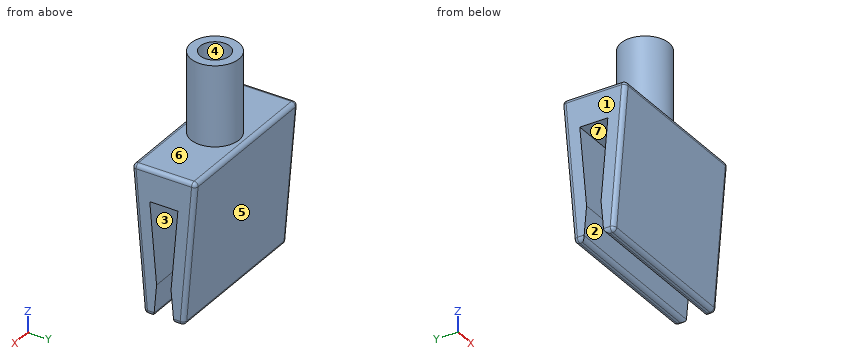
```python
from build123d import *

# Parameters (mm, degrees)
F1_DEPTH = 10
F3_DEPTH = 25
F4_R     = 0.5
F5_R     = 3
F5_R_2   = 1.85
F6_DEPTH = 10


with BuildPart() as f1:
    # F0 (on Right) → F1 (new body, symmetric)
    with BuildSketch(Plane.YZ):
        Polygon((-45.5818854975, 27.2887923438), (-44.0818854975, 9.2887923438), (-39.0818854975, 9.2887923438), (-37.5818854975, 27.2887923438), align=None)
    extrude(amount=F1_DEPTH, both=True)

    # F2 (on face) → F3 (cut)
    with BuildSketch(Plane.YZ.offset(10)):
        Polygon((-42.8318854975, 9.2887923438), (-40.3318854975, 9.2887923438), (-40.6818854975, 13.2887923438), (-39.8318854975, 23.2887923438), (-41.5818854975, 23.2887923438), (-43.3318854975, 23.2887923438), (-42.4818854975, 13.2887923438), align=None)
    extrude(amount=-F3_DEPTH, mode=Mode.SUBTRACT)

    # F4
    f4_edges = [f1.edges().sort_by_distance(p)[0] for p in [
        (10, -44.831885, 18.288792),
        (10, -41.581885, 27.288792),
        (10, -38.331885, 18.288792),
        (0, -39.081885, 9.288792),
        (0, -44.081885, 9.288792),
        (-10, -44.831885, 18.288792),
        (-10, -38.331885, 18.288792),
        (0, -37.581885, 27.288792),
        (0, -45.581885, 27.288792),
        (-10, -41.581885, 27.288792),
        (-10, -39.706885, 9.288792),
        (0, -40.331885, 9.288792),
        (-10, -43.456885, 9.288792),
        (0, -42.831885, 9.288792),
        (10, -39.706885, 9.288792),
        (10, -43.456885, 9.288792),
    ]]
    fillet(f4_edges, radius=F4_R)

    # F5 (on face) → F6 (join)
    with BuildSketch(Plane.XY.offset(27.2887923438)):
        with Locations((0, -41.5818854975)):
            Circle(F5_R)
        with Locations((0, -41.5818854975)):
            Circle(F5_R_2, mode=Mode.SUBTRACT)
    extrude(amount=F6_DEPTH)


solid = f1.part
```
Could you check a few things on this model? Use its own coordinates, in mm. Face numbers are marked on the shaded views. A direction names the side the tool comes from. Round coordinates to 2 decimals unless told otherwise and drop trailing zeros. Write each loop counter-clockwise with the first axis right and the second up, starting at its lowest first coordinate (ties: lowest second). Pieces come first, ordered by that corner, then holes. Notation, with made-up numbers: M 10,34.25 L 22,34.25 A28 ccw 22,71.25 Z; hole C 35,-21.5 d2. An arc over 180 degrees is marked long. Write each question's results on one line, items separated by ' | '. Start each with the question number.
1. Thinking about a two-plate mould opening in Y: for the marked faces 5, 6 and 7, which applies, +Y half, -Y half, draft (parallel to the pull), parting line (faces both ways), or undercut?
2. Imagine slicing it at A-A on x = 0. List the corners of the cut face in (y, z) for me.
3. I need wall thicknesses on L1, parallel to Y at x = 0, z = 32.75; L2, parallel to Z at x = 7, y = -41.25; L3, parallel to X at y = -38.5, z = 21.25. Which ranges of each line are inside material? Lowest first, please. Write a range as from..to.
4. On a 3-axis mill with a long thin cutter (end or side, diameter ignored), from which of +Z, -Z, +X, -X, +Y, -Y can I reach the whole of each face in a straight line? I mean the marked faces 1, 2, 3 and 4. Say none if no direction works.
5. I'm going to push flat-ended pins straight in: pin 1 Ø1.5 at (x, y) = (7.5, -43) entering from -Z; pin 2 Ø1 at (x, z) = (3, 31.5) entering from -Y; pin 3 Ø1 at (x, y) = (-2, -41.5) entering from -Z; pin 4 Ø3 at (x, z) = (4, 23) entering from -Y. Where does each tip first touch, or does it pass through?
6. Imagine slicing it at B-B on y = -42. List the corners of the cut face in (x, z) for me, and give its area (3 significant figures).
7. Imagine slicing it at D-D on z = 34. List the corners of the cut face in (x, y) for me.
8. Imagine slicing it at C-C on x = -8.25. List the corners of the cut face in (y, z) for me.
Result sheet:
1) face 5: +Y half | face 6: draft | face 7: undercut
2) outline: M -45.54,26.75 L -44.12,9.75 A0.5 ccw -43.62,9.29 L -43.29,9.29 A0.5 ccw -42.79,9.75 L -42.48,13.29 L -43.33,23.29 L -39.83,23.29 L -40.68,13.29 L -40.37,9.75 A0.5 ccw -39.87,9.29 L -39.54,9.29 A0.5 ccw -39.04,9.75 L -37.63,26.75 A0.5 ccw -38.13,27.29 L -38.58,27.29 L -38.58,37.29 L -39.73,37.29 L -39.73,27.29 L -43.43,27.29 L -43.43,37.29 L -44.58,37.29 L -44.58,27.29 L -45.04,27.29 A0.5 ccw Z
3) L1: y = -44.58..-43.43, -39.73..-38.58 | L2: z = 23.29..27.29 | L3: x = -9.99..9.99
4) face 1: +Z, -Z, -X, +Y, -Y | face 2: -Z, +X, -X | face 3: +X, -X | face 4: +Z
5) pin 1: stops at z = 9.29 | pin 2: stops at y = -43.24 | pin 3: stops at z = 23.29 | pin 4: stops at y = -45.35
6) outline: M -10,23.29 L 10,23.29 L 10,26.79 A0.5 ccw 9.5,27.29 L 2.97,27.29 L 2.97,37.29 L 1.8,37.29 L 1.8,27.29 L -1.8,27.29 L -1.8,37.29 L -2.97,37.29 L -2.97,27.29 L -9.5,27.29 A0.5 ccw -10,26.79 Z | area: 103 mm^2
7) outline: C 0,-41.58 d6; hole C 0,-41.58 d3.7
8) outline: M -45.54,26.75 L -44.12,9.75 A0.5 ccw -43.62,9.29 L -43.29,9.29 A0.5 ccw -42.79,9.75 L -42.48,13.29 L -43.33,23.29 L -39.83,23.29 L -40.68,13.29 L -40.37,9.75 A0.5 ccw -39.87,9.29 L -39.54,9.29 A0.5 ccw -39.04,9.75 L -37.63,26.75 A0.5 ccw -38.13,27.29 L -45.04,27.29 A0.5 ccw Z
